Geometry check sheet. Reference: the model listing, model coordinates, mm. Round coordinates to 2 decimals unless told otherwise and drop trailing zeros. Write each loop counter-clockwise with the first axis right and the second up, starting at its lowest first coordinate (ties: lowest second). Pieces come first, ordered by that corner, then holes. Notation, with made-up numbers: (15.25, -19.75) -> (30.25, -19.75) arc R15 cw to (30.25, -1.75) -> close; hole circle Ø5 at (37, 73). An arc over 180 degrees is marked (long way). Use a Markdown table: item, result.
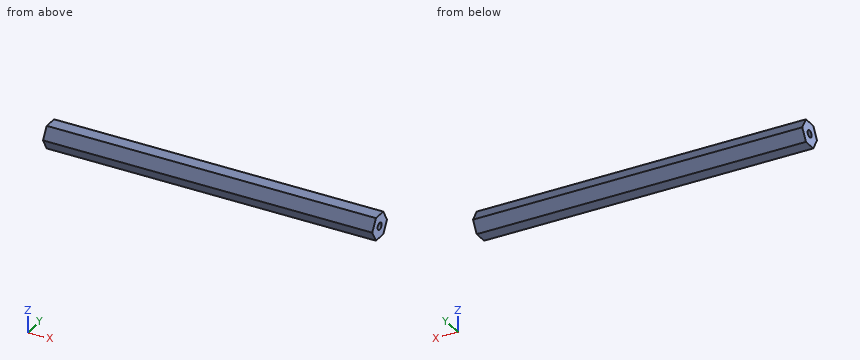
Autodesk Inventor part; units mm, degrees
ref_plane "YZ Plane" through (0, 0, 0) normal (1, 0, 0) x (0, 1, 0)
ref_plane "XZ Plane" through (0, 0, 0) normal (0, 1, 0) x (-1, 0, 0)
ref_plane "XY Plane" through (0, 0, 0) normal (0, 0, 1) x (1, 0, 0)
sketch "Sketch1" plane through (0, 0, 0) normal (1, 0, 0) x (0, 1, 0)
  line L0 (-3.6662, -6.35) -> (-7.3323, 0)
  line L1 (-7.3323, 0) -> (-3.6662, 6.35)
  line L2 (-3.6662, 6.35) -> (3.6662, 6.35)
  line L3 (3.6662, 6.35) -> (7.3323, 0)
  line L4 (7.3323, 0) -> (3.6662, -6.35)
  line L5 (3.6662, -6.35) -> (-3.6662, -6.35)
  point P0 (0, 0)
  point P1 (0, 0)
  dimension "d0" = 12.7
extrude "Extrusion1" add sketch "Sketch1" along normal blind 184.023
sketch "Sketch2" plane through (184.023, 0, 0) normal (1, 0, 0) x (0, 0, -1)
  point P0 (0, 0)
  point P1 (0, 0)
hole "Hole1" at (184.023, 0, 0) direction (-1, 0, 0) diameter 3.9624 depth 31.75 tip angle 118
sketch "Sketch3" plane through (0, 0, 0) normal (-1, 0, 0) x (0, 0, 1)
  circle A0 centre (0, 0) radius 1.9812
hole "Hole2" at (0, 0, 0) direction (1, 0, 0) diameter 3.9624 depth 31.75 tip angle 118
properties part number "STOCK,HEX,SHAFT,KICKER,FRONT" material "Aluminum 6061"
(1) Section check A-A on x = 20. Record the cut outline in (y, z), plus the area to 3 significant figures.
A:
| item | result |
|---|---|
| outline | (-7.33, 0) -> (-3.67, -6.35) -> (3.67, -6.35) -> (7.33, 0) -> (3.67, 6.35) -> (-3.67, 6.35) -> close; hole circle Ø3.96 at (0, 0) |
| area | 127 mm2 |
(2) Thickness scan on line 1 (Z direction, x = 175, y = 0); line 2 (Y direction, x = 162, z = 0); line 3 (Y direction, x = 142, z = -1.75). Record the ranges inside material, lowest first.
A:
| item | result |
|---|---|
| line 1 | z = -6.35 to -1.98, 1.98 to 6.35 |
| line 2 | y = -7.33 to -1.98, 1.98 to 7.33 |
| line 3 | y = -6.32 to 6.32 |
(3) Section check B-B on x = 100. Record the cut outline in (y, z), plus the area to 3 significant figures.
A:
| item | result |
|---|---|
| outline | (-7.33, 0) -> (-3.67, -6.35) -> (3.67, -6.35) -> (7.33, 0) -> (3.67, 6.35) -> (-3.67, 6.35) -> close |
| area | 140 mm2 |
(4) Section check C-C on z = -3.5. Record the cut outline in (x, y).
A:
| item | result |
|---|---|
| outline | (0, -5.31) -> (184.02, -5.31) -> (184.02, 5.31) -> (0, 5.31) -> close |
(5) Gauge pin test, flat ends, axial feed: pin 1 Ø3.5 at (y, z) = (0, 0) entering from -X; pin 2 Ø3 at (x, z) = (129, 4.5) entering from +Y. Record the tip position at first contact, or that the pin passes through.
A:
| item | result |
|---|---|
| pin 1 | stops at x = 31.89 |
| pin 2 | stops at y = 5.6 |
